Check sheet for the modelled part. Datum: model origin and axes. Units: mm. A direction names the side the tool comes from. Give positions to 0.01 mm unless a question says otherwise; leave off trailing zeros. Order: outer loops, then holes, each group sorted by start corner. A loop starts at its lowest first (then second) coordinate and runs counter-clockwise, first axis right, second up. Notation, with made-up numbers: (44, -34.75) -> (49, -34.75) arc R12 cw to (49, -25.75) -> close; hole circle Ø11 at (-5.75, 85.25). An arc over 180 degrees is marked (long way). Answer in a Markdown table with one row per item. Add a question column.
(1) Cross-section at C-C (y = -37). Record the cut outline in (x, z).
(2) Thickness scan on L1, parallel to Z at x = 40.5, y = 19; L2, parallel to Y at x = 0, z = -48; L3, parallel to Y at x = 0, z = -55.5. Record the ranges inside material, lowest first. Write a range as [from, to].
(3) Cross-section at D-D (y = 59). Record the cut outline in (x, z).
(4) Set-up check for faces 4 (the face through (-25, 38, -3)), 5 (the face through (30, 5, -48.6)), 6 (the face through (11.5, 22.2, -43)), 7 (the face through (-31, -25, -19)), 8 (the face through (-12, -25, -52)): record each of +Z, -Z, +X, -X, +Y, -Y from which the full face is reachable in a straight line by a thin tool's end or side.
(5) Release check for a two-part mould opening along Z. For faces 1 (the face through (25, -24, -34)), 2 (the face through (-37.675, 5.734, -51.657)), 3 (the face through (-23, 0, -54.8)) record: released by +Z, released by -Z, zero draft, split by the parting line, or undercut.
(6) Cross-section at A-A (z = -52). Record the cut outline in (x, y).
(7) Go/stop test with flat-tipped pins: pin 1 (15 mm diameter, centred on x = 56, y = -8.5, fed in from -Z); pin 2 (6 mm diameter, centred on x = 43.5, z = -4.5, fed in from -Y); pin 3 (25 mm diameter, centred on x = 0.5, y = 42, fed in from -Z); pin 4 (7 mm diameter, centred on y = 38.5, z = -2.5, fed in from -X). Record where each tip stops, or that it passes through.
(8) Cross-section at B-B (x = -40.5). Record the cut outline in (y, z).
```python
from build123d import *

# Parameters (mm, degrees)
F1_DEPTH  = 6.2
F3_DEPTH  = 6.2
F5_DEPTH  = 10
F7_DEPTH  = 6.2
F9_DEPTH  = 9
F11_DEPTH = 6.2
F13_DEPTH = 11
F15_DEPTH = 6.2
F16_R     = 22.25
F17_DEPTH = 13
F19_D     = 35
F19_DEPTH = 35
F19_TIP   = 10.515060833


# Not quite as in the source:
# - a feature names something its author has since deleted; it is built from what else it names


with BuildPart() as f1:
    # F0 (on Top) → F1 (new body)
    with BuildSketch(Plane.XY):
        Polygon((11.0905365064, -25), (25, -25), (102, 13), (102, 25), (11.0905365064, 25), (-11.0905365064, 25), (-25, 25), (-102, -13), (-102, -25), (-11.0905365064, -25), align=None)
    extrude(amount=F1_DEPTH)

    # F2 (on face) → F3 (join)
    with BuildSketch(Plane(origin=(0, 0, 0), x_dir=(1, 0, 0), z_dir=(0, 0, -1))):
        Polygon((-25, 25), (-25, 0), (-25, -25), (25, -25), (25, 0), (25, 25), align=None)
        Polygon((25, -25), (-25, -25), (-25, -102), (-13, -102), align=None)
        Polygon((13, 102), (-25, 25), (25, 25), (25, 102), align=None)
    extrude(amount=F3_DEPTH)

    # F4 (on face) → F5 (join)
    with BuildSketch(Plane(origin=(0, 0, -6.2), x_dir=(1, 0, 0), z_dir=(0, 0, -1))):
        with BuildLine():
            ThreePointArc((-25, 2.61e-08), (-1.3e-08, -25), (25, 0))
            ThreePointArc((25, 0), (1.3e-08, 25), (-25, 2.61e-08))
        make_face()
    extrude(amount=F5_DEPTH)

    # F6 (on face) → F7 (join)
    with BuildSketch(Plane(origin=(0, 0, -16.2), x_dir=(1, 0, 0), z_dir=(0, 0, -1))):
        with BuildLine():
            Line((-5.83e-08, -25), (25, -25))
            Line((25, -25), (25, 0))
            ThreePointArc((25, 0), (17.677669509, -17.6776695503), (-5.83e-08, -25))
        make_face()
        with BuildLine():
            Line((-25, -25), (-5.83e-08, -25))
            ThreePointArc((-5.83e-08, -25), (-17.6776695503, -17.677669509), (-25, 0))
            Line((-25, 0), (-25, -25))
        make_face()
        Polygon((25, 0), (25, -25), (88, -25), (88, -13), (25, 25), align=None)
        Polygon((-88, 13), (-25, -25), (-25, 0), (-25, 25), (-88, 25), align=None)
        with BuildLine():
            ThreePointArc((-25, 0), (-17.6776695503, -17.677669509), (-5.83e-08, -25))
            ThreePointArc((-5.83e-08, -25), (17.677669509, -17.6776695503), (25, 0))
            ThreePointArc((25, 0), (17.6776695297, 17.6776695297), (0, 25))
            ThreePointArc((0, 25), (-17.6776695297, 17.6776695297), (-25, 0))
        make_face()
        with BuildLine():
            Line((-25, 25), (-25, 0))
            ThreePointArc((-25, 0), (-17.6776695297, 17.6776695297), (0, 25))
            Line((0, 25), (-25, 25))
        make_face()
        with BuildLine():
            ThreePointArc((0, 25), (17.6776695297, 17.6776695297), (25, 0))
            Line((25, 0), (25, 25))
            Line((25, 25), (0, 25))
        make_face()
    extrude(amount=F7_DEPTH)

    # F8 (on face) → F9 (join)
    with BuildSketch(Plane(origin=(0, 0, -22.4), x_dir=(1, 0, 0), z_dir=(0, 0, -1))):
        with BuildLine():
            ThreePointArc((-5.83e-08, -25), (17.677669509, -17.6776695503), (25, 0))
            ThreePointArc((25, 0), (17.6776695297, 17.6776695297), (0, 25))
            ThreePointArc((0, 25), (-25, 2.92e-08), (-5.83e-08, -25))
        make_face()
    extrude(amount=F9_DEPTH)

    # F10 (on face) → F11 (join)
    with BuildSketch(Plane(origin=(0, 0, -31.4), x_dir=(1, 0, 0), z_dir=(0, 0, -1))):
        Polygon((13, 75), (-25, 25), (4.22e-08, 25), (25, 25), (25, 75), align=None)
        with BuildLine():
            ThreePointArc((4.22e-08, 25), (17.6776695446, 17.6776695147), (25, 0))
            Line((25, 0), (25, 25))
            Line((25, 25), (4.22e-08, 25))
        make_face()
        with BuildLine():
            ThreePointArc((-25, 0), (-17.6776695332, -17.6776695262), (-9.9e-09, -25))
            ThreePointArc((-9.9e-09, -25), (17.6776695262, -17.6776695332), (25, 0))
            ThreePointArc((25, 0), (17.6776695446, 17.6776695147), (4.22e-08, 25))
            ThreePointArc((4.22e-08, 25), (-17.6776695147, 17.6776695446), (-25, 0))
        make_face()
        with BuildLine():
            ThreePointArc((25, 0), (17.6776695262, -17.6776695332), (-9.9e-09, -25))
            Line((-9.9e-09, -25), (25, -25))
            Line((25, -25), (25, 0))
        make_face()
        Polygon((-9.9e-09, -25), (-25, -25), (-25, -75), (-13, -75), (25, -25), align=None)
        with BuildLine():
            Line((-25, 0), (-25, -25))
            Line((-25, -25), (-9.9e-09, -25))
            ThreePointArc((-9.9e-09, -25), (-17.6776695332, -17.6776695262), (-25, 0))
        make_face()
        with BuildLine():
            Line((-25, 25), (-25, 0))
            ThreePointArc((-25, 0), (-17.6776695147, 17.6776695446), (4.22e-08, 25))
            Line((4.22e-08, 25), (-25, 25))
        make_face()
    extrude(amount=F11_DEPTH)

    # F12 (on face) → F13 (join)
    with BuildSketch(Plane(origin=(0, 0, -37.6), x_dir=(1, 0, 0), z_dir=(0, 0, -1))):
        with BuildLine():
            ThreePointArc((-25, 2.61e-08), (-1.3e-08, -25), (25, 0))
            ThreePointArc((25, 0), (1.3e-08, 25), (-25, 2.61e-08))
        make_face()
    extrude(amount=F13_DEPTH)

    # F14 (on face) → F15 (join)
    with BuildSketch(Plane(origin=(0, 0, -48.6), x_dir=(1, 0, 0), z_dir=(0, 0, -1))):
        with BuildLine():
            ThreePointArc((-25, 0), (-17.6776695204, -17.6776695389), (2.61e-08, -25))
            ThreePointArc((2.61e-08, -25), (17.6776695389, -17.6776695204), (25, 0))
            ThreePointArc((25, 0), (17.6776695389, 17.6776695204), (2.61e-08, 25))
            ThreePointArc((2.61e-08, 25), (-17.6776695204, 17.6776695389), (-25, 0))
        make_face()
        with BuildLine():
            ThreePointArc((2.61e-08, 25), (17.6776695389, 17.6776695204), (25, 0))
            Line((25, 0), (25, 25))
            Line((25, 25), (2.61e-08, 25))
        make_face()
        with BuildLine():
            Line((2.61e-08, -25), (25, -25))
            Line((25, -25), (25, 0))
            ThreePointArc((25, 0), (17.6776695389, -17.6776695204), (2.61e-08, -25))
        make_face()
        with BuildLine():
            Line((-25, -25), (2.61e-08, -25))
            ThreePointArc((2.61e-08, -25), (-17.6776695204, -17.6776695389), (-25, 0))
            Line((-25, 0), (-25, -25))
        make_face()
        with BuildLine():
            Line((-25, 25), (-25, 0))
            ThreePointArc((-25, 0), (-17.6776695204, 17.6776695389), (2.61e-08, 25))
            Line((2.61e-08, 25), (-25, 25))
        make_face()
        Polygon((-50, 13), (-25, -25), (-25, 0), (-25, 25), (-50, 25), align=None)
        Polygon((25, 0), (25, -25), (50, -25), (50, -13), (25, 25), align=None)
    extrude(amount=F15_DEPTH)

    # F16 (on face) → F17 (join)
    with BuildSketch(Plane(origin=(0, 0, -54.8), x_dir=(1, 0, 0), z_dir=(0, 0, -1))):
        Circle(F16_R)
    extrude(amount=F17_DEPTH)

    # F19
    with Locations(Plane(origin=(0, 0, -67.8), x_dir=(1, 0, 0), z_dir=(0, 0, -1))):
        with Locations((0, 0)):
            Hole(F19_D / 2, depth=F19_DEPTH)
            with Locations((0, 0, -(F19_DEPTH + F19_TIP / 2))):  # 118° drill point
                Cone(0, F19_D / 2, F19_TIP, mode=Mode.SUBTRACT)


solid = f1.part
```
Answer below:
| question | item | result |
|---|---|---|
| 1 | outline | (-19.08, -6.2) -> (25, -6.2) -> (25, 0) -> (-19.08, 0) -> close; (-15.88, -37.6) -> (25, -37.6) -> (25, -31.4) -> (-15.88, -31.4) -> close |
| 2 | L1 | z = [-54.8, -48.6], [-22.4, -16.2], [0, 6.2] |
| 2 | L2 | y = [-25, -17.5], [17.5, 25] |
| 2 | L3 | y = [-22.25, -17.5], [17.5, 22.25] |
| 3 | outline | (-25, -37.6) -> (-0.84, -37.6) -> (-0.84, -31.4) -> (-25, -31.4) -> close; (-25, -6.2) -> (8.22, -6.2) -> (8.22, 0) -> (-25, 0) -> close |
| 4 | face 4 | -X, +Y, -Y |
| 4 | face 5 | +X |
| 4 | face 6 | none |
| 4 | face 7 | +X, -X, -Y |
| 4 | face 8 | -Z, +X, -X, -Y |
| 5 | face 1 | undercut |
| 5 | face 2 | zero draft |
| 5 | face 3 | released by -Z |
| 6 | outline | (-50, -25) -> (25, -25) -> (50, 13) -> (50, 25) -> (-25, 25) -> (-50, -13) -> close; hole circle Ø35 at (0, 0) |
| 7 | pin 1 | stops at z = -22.4 |
| 7 | pin 2 | passes through |
| 7 | pin 3 | stops at z = -37.6 |
| 7 | pin 4 | stops at x = -25 |
| 8 | outline | (-25, -54.8) -> (1.44, -54.8) -> (1.44, -48.6) -> (-25, -48.6) -> close; (-25, -22.4) -> (15.65, -22.4) -> (15.65, -16.2) -> (-25, -16.2) -> close; (-25, 0) -> (17.35, 0) -> (17.35, 6.2) -> (-25, 6.2) -> close |
